Work out the finished part from the listing and answer in its coordinate system (mm). Give positions to 0.01 mm unless a question says otherwise; leave off trailing zeros. Write each loop counter-clockwise with the first axis right and the second up, starting at its lowest first coordinate (ties: lowest second). Pieces come first, ordered by that corner, then holes. Notation, with made-up numbers: (6.5, 53.25) -> (40.5, 53.25) arc R21 cw to (40.5, 62.25) -> close; hole circle Ø5 at (66, 35.25). An arc over 180 degrees is marked (long way). Use a Markdown table: item, result. Add a question column.
Q1. Consider line 1 (X direction, y = -0.25, z = 257.5); line 2 (Y direction, x = -2, z = 23); line 3 (Z direction, x = -3.75, y = -3.25). Determine where each line is inside the solid, lowest interval first.
Q2. Section A-A, the plane z = 304 is taken. Give the vertices of the cut face in (x, y), plus the area to 3 significant figures.
Q3. Each of these flat-tipped pins is pushed along its axis until it touches: pin 1 Ø2 at (y, z) = (-2, 257) entering from +X; pin 2 Ø1.5 at (x, y) = (3.5, 2) entering from -Z. Where does it stop, or does it pass through?
from build123d import *

# Parameters (mm, degrees)
SKETCH1_R           = 5
BOSS_EXTRUDE1_DEPTH = 465
CHAMFER1_SIZE       = 0.5
CHAMFER2_SIZE       = 0.5


with BuildPart() as part:
    # Sketch1 → Boss-Extrude1 (new body)
    with BuildSketch(Plane.XY):
        Circle(SKETCH1_R)
    extrude(amount=BOSS_EXTRUDE1_DEPTH)

    # Chamfer1
    chamfer1_edges = [part.edges().sort_by_distance(p)[0] for p in [
        (-5, 0, 465),
    ]]
    chamfer(chamfer1_edges, length=CHAMFER1_SIZE)

    # Chamfer2
    chamfer2_edges = [part.edges().sort_by_distance(p)[0] for p in [
        (-5, 0, 0),
    ]]
    chamfer(chamfer2_edges, length=CHAMFER2_SIZE)


solid = part.part
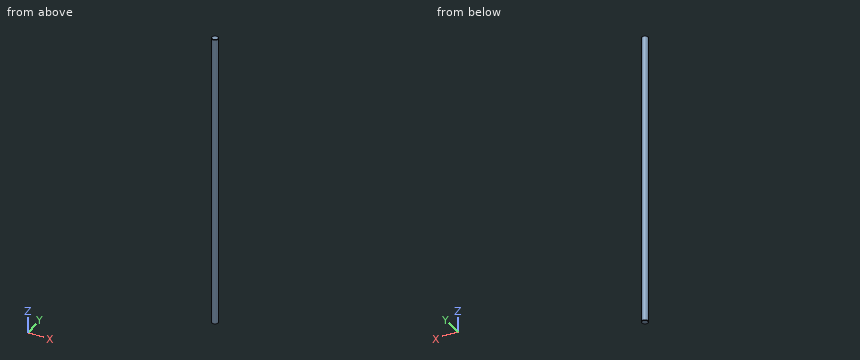
Result set:
| question | item | result |
|---|---|---|
| 1 | line 1 | x = -4.99 to 4.99 |
| 1 | line 2 | y = -4.58 to 4.58 |
| 1 | line 3 | z = 0.46 to 464.54 |
| 2 | outline | circle Ø10 at (0, 0) |
| 2 | area | 78.5 mm2 |
| 3 | pin 1 | stops at x = 4.9 |
| 3 | pin 2 | stops at z = 0 |
